Autodesk Inventor part; units mm, degrees
ref_plane "YZ Plane" through (0, 0, 0) normal (1, 0, 0) x (0, 1, 0)
ref_plane "XZ Plane" through (0, 0, 0) normal (0, 1, 0) x (-1, 0, 0)
ref_plane "XY Plane" through (0, 0, 0) normal (0, 0, 1) x (1, 0, 0)
sketch "Sketch1" plane through (0, 0, 0) normal (0, 0, 1) x (1, 0, 0)
  arc A0 (23.9202, -3.175) -> (23.9202, 3.175) centre (0, 0) ccw
  line L0 (23.9202, 3.175) -> (150.9202, 3.175)
  line L1 (150.9202, 3.175) -> (150.9202, -3.175)
  line L2 (150.9202, -3.175) -> (23.9202, -3.175)
  line L3 (23.9202, 3.175) -> (0, 3.175) construction
  line L4 (0, 0) -> (0, 3.175) construction
  line L5 (0, 0) -> (0, -3.175) construction
  line L6 (0, -3.175) -> (23.9202, -3.175) construction
  dimension "d0" = 24.13
  dimension "d1" = 6.35
  dimension "d9" = 127
extrude "Extrusion1" add sketch "Sketch1" along normal blind 177.8
sketch "Sketch2" plane through (23.9202, 3.175, 0) normal (0, 1, 0) x (1, 0, 0)
  line L0 (0, -177.8) -> (127, -177.8)
  line L1 (127, 0) -> (127, -177.8)
  line L2 (0, 0) -> (127, 0)
  line L3 (127, -50.8) -> (38.1, -50.8)
  line L4 (38.1, -50.8) -> (38.1, -127)
  line L5 (38.1, -127) -> (127, -127)
  line L6 (127, -127) -> (127, -50.8)
  line L7 (38.1, -50.8) -> (38.1, 0) construction
  line L8 (38.1, -127) -> (38.1, -177.8) construction
  line L9 (0, 0) -> (0, -177.8)
  point P0 (-23.9202, 0)
  dimension "d4" = 76.2
  dimension "d8" = 38.1
extrude "Extrusion2" cut sketch "Sketch2" against normal up to next contours L5 L4 L3 L1
properties part number "PitchingArmConcept"
Geometry check sheet. Reference: the model listing, model coordinates, mm. A direction names the side the tool comes from. Round coordinates to 2 decimals unless told otherwise and drop trailing zeros. Write each loop counter-clockwise with the first axis right and the second up, starting at its lowest first coordinate (ties: lowest second). Pieces come first, ordered by that corner, then holes. Notation, with made-up numbers: (-27.75, 40.25) - (7.25, 40.25) arc R9 cw to (7.25, 56.25) - close; hole circle Ø1 at (37, 10). An arc over 180 degrees is marked (long way). One line per item, written item: value.
1. Mould release check, pull along Z, two halves, no side actions. Record for faces 1 (the face through (62.02, 0, 88)), 2 (the face through (87, 0, 0)), 3 (the face through (60, -3.175, 88)): released by +Z, released by -Z, zero draft, split by the parting line, or undercut.
The answers:
face 1: undercut
face 2: released by -Z
face 3: zero draft
2. Set-up check for faces 4 (the face through (107, 0, 50.8)), 5 (the face through (87, 0, 177.8)): record each of +Z, -Z, +X, -X, +Y, -Y from which the full face is reachable in a straight line by a thin tool's end or side.
The answers:
face 4: +X, +Y, -Y
face 5: +Z, +X, -X, +Y, -Y
3. Cross-section at A-A on x = 80.5. Record the boundary of the cut face in (y, z) (3 decimals).
The answers:
outline: (-3.175, 0) - (3.175, 0) - (3.175, 50.8) - (-3.175, 50.8) - close; (-3.175, 127) - (3.175, 127) - (3.175, 177.8) - (-3.175, 177.8) - close
4. Scan lines: L1, parallel to Z at x = 114, y = -0.25; L2, parallel to X at y = 1, z = 52; L3, parallel to X at y = -1.25, z = 46.5. Record each from-to range of solid material in increasing order.
The answers:
L1: z = 0 to 50.8, 127 to 177.8
L2: x = 24.11 to 62.02
L3: x = 24.1 to 150.92
5. Cross-section at C-C on z = 86. Record the boundary of the cut face in (x, y) (3 decimals).
The answers:
outline: (23.92, -3.175) - (62.02, -3.175) - (62.02, 3.175) - (23.92, 3.175) arc R24.13 cw to start
6. Depth check by flat-ended pin: pin 1 Ø3 at (y, z) = (-1, 105.5) entering from -X. Enter the tip coordinate at first touch or a pass-through.
The answers:
pin 1: stops at x = 24
7. Cross-section at B-B on y = -0.75. Record the boundary of the cut face in (x, z), and give its area (3 significant figures).
The answers:
outline: (24.12, 0) - (150.92, 0) - (150.92, 50.8) - (62.02, 50.8) - (62.02, 127) - (150.92, 127) - (150.92, 177.8) - (24.12, 177.8) - close
area: 15,800 mm^2
